Work out the finished part from the listing and answer in its coordinate system (mm). A direction names the side the tool comes from. Round coordinates to 2 decimals unless told otherwise and drop trailing zeros. Loops run counter-clockwise (first coordinate to the right, second up) from the corner with the lowest first, then second, coordinate; pieces in that order, holes last. Notation, with made-up numbers: (26, 61) -> (45, 61) arc R21 cw to (45, 95) -> close; hole circle Ø11 at (77, -22). An arc over 180 degrees is marked (long way). Use one line per item in the form item = value.
```python
from build123d import *

# Parameters (mm, degrees)
F1_DEPTH = 57.15
F2_R     = 12.7
F3_DEPTH = 44.45
F4_R     = 5.08
F5_DEPTH = 13.7758108493


# Not quite as in the source:
# - ends of sketch curves that miss each other by under 0.0002 mm in the source are joined


with BuildPart() as f1:
    # F0 (on Front) → F1 (new body)
    with BuildSketch(Plane.XZ):
        Polygon((-31.75, 0), (31.75, 0), (31.75, 12.7), (13.4683688998, 12.7), (13.4683688998, 21.59), (63.5, 21.59), (63.5, 85.09), (-63.5, 85.09), (-63.5, 21.59), (-13.4683688998, 21.59), (-13.4683688998, 12.7), (-31.75, 12.7), align=None)
    extrude(amount=-F1_DEPTH)

    # F2 (on face) → F3 (cut)
    with BuildSketch(Plane.XZ):
        with BuildLine():
            Line((0, 85.09), (-63.5, 85.09))
            Line((-63.5, 85.09), (-63.5, 34.29))
            Line((-63.5, 34.29), (-47.625, 34.29))
            Line((-47.625, 34.29), (-21.0934436414, 73.8401851094))
            ThreePointArc((-21.0934436414, 73.8401851094), (-11.9529513968, 82.101783869), (0, 85.09))
        make_face()
        with Locations((0, 59.69)):
            Circle(F2_R)
        with BuildLine():
            Line((63.5, 85.09), (0, 85.09))
            ThreePointArc((0, 85.09), (11.9529513968, 82.101783869), (21.0934436414, 73.8401851094))
            Line((21.0934436414, 73.8401851094), (47.625, 34.29))
            Line((47.625, 34.29), (63.5, 34.29))
            Line((63.5, 34.29), (63.5, 85.09))
        make_face()
    extrude(amount=-F3_DEPTH, mode=Mode.SUBTRACT)

    # F4 (on face) → F5 (cut, through all)
    with BuildSketch(Plane.XY.offset(85.09)):
        with Locations((-0.0332157188, 22.225)):
            Circle(F4_R)
    extrude(amount=-F5_DEPTH, mode=Mode.SUBTRACT)


solid = f1.part
```
(1) Find section A-A, the plane y = 37. Write down the section's boundary in (x, z) (3 decimals), then the cut area to 3 significant figures.
Completed:
outline = (-63.5, 21.59) -> (-13.468, 21.59) -> (-13.468, 12.7) -> (-31.75, 12.7) -> (-31.75, 0) -> (31.75, 0) -> (31.75, 12.7) -> (13.468, 12.7) -> (13.468, 21.59) -> (63.5, 21.59) -> (63.5, 34.29) -> (47.625, 34.29) -> (21.093, 73.84) arc R25.4 ccw to (0, 85.09) arc R25.4 ccw to (-21.093, 73.84) -> (-47.625, 34.29) -> (-63.5, 34.29) -> close; hole circle Ø25.4 at (0, 59.69)
area = 5,200 mm2
(2) For a pull along Z with two mould halves and no side action, classify faces 1 (the flat face through (45, 44.45, 66)), 2 (the flat face through (1, 51, 85.09)), 3 (the flat face through (-13.468, 28, 17)) as +Z half, -Z half, draft (parallel to the pull), parting line (faces both ways), or undercut.
Completed:
face_1 = draft
face_2 = +Z half
face_3 = undercut
(3) Find section B-B, the plane x = -3.5. Write down the section's boundary in (y, z).
Completed:
outline = (0, 0) -> (57.15, 0) -> (57.15, 85.09) -> (44.45, 85.09) -> (44.45, 84.85) -> (25.94, 84.85) -> (25.94, 71.9) -> (44.45, 71.9) -> (44.45, 47.48) -> (0, 47.48) -> close; (0, 71.9) -> (18.51, 71.9) -> (18.51, 84.85) -> (0, 84.85) -> close
(4) Consider L1, parallel to Z at x = 0, y = 34; L2, parallel to Z at x = -24, y = 48; L3, parallel to Y at x = -22, z = 80. Determine where each line is inside the solid, lowest interval first.
Completed:
L1 = 0 to 46.99, 72.39 to 85.09
L2 = 0 to 12.7, 21.59 to 85.09
L3 = 44.45 to 57.15
(5) Find section D-D, the plane z = 78. Write down the section's boundary in (x, y) (3 decimals).
Completed:
outline = (-63.5, 44.45) -> (-17.604, 44.45) -> (-17.604, 0) -> (17.604, 0) -> (17.604, 44.45) -> (63.5, 44.45) -> (63.5, 57.15) -> (-63.5, 57.15) -> close; hole circle Ø10.16 at (-0.033, 22.225)
(6) Given P1, Ø1.5, axis at y = 10, z = 45.5, coming from the -X side; P2, Ø8, axis at x = 44, y = 15.5, coming from the -Z side; P3, Ø9, axis at x = 22.5, y = 23.5, coming from the +Z side, each flat-ended and moving along its own axis, determine where each tip first touches the part or whether it passes through.
Completed:
P1 = -40.61
P2 = 21.59
P3 = 77.61
(7) For faces 4 (the flat face through (-56, 22, 34.29)), 5 (the flat face through (-39, 28, 21.59)), 6 (the flat face through (31.75, 28, 6)), 7 (the cylindrical face through (-0.695, 27.262, 78.299)), 8 (the flat face through (38, 28, 21.59)), determine the directions among +Z, -Z, +X, -X, +Y, -Y from which every point of the face is accessible in a straight line to the end or side of a thin tool.
Completed:
face_4 = +Z, -X, -Y
face_5 = -X, +Y, -Y
face_6 = -Z, +X, +Y, -Y
face_7 = +Z
face_8 = +X, +Y, -Y
(8) Find section C-C, the plane y = 47. Write down the section's boundary in (x, z), then the cut area to 3 significant figures.
Completed:
outline = (-63.5, 21.59) -> (-13.47, 21.59) -> (-13.47, 12.7) -> (-31.75, 12.7) -> (-31.75, 0) -> (31.75, 0) -> (31.75, 12.7) -> (13.47, 12.7) -> (13.47, 21.59) -> (63.5, 21.59) -> (63.5, 85.09) -> (-63.5, 85.09) -> close
area = 9,110 mm2
